For this review, take the finished solid that the model builds, in its own axes (mm). Round coordinates to 2 decimals unless told otherwise and drop trailing zeros. Order: outer loops, then holes, each group sorted by start corner. A loop starts at its lowest first (then second) coordinate and runs counter-clockwise, first axis right, second up. Notation, with made-up numbers: M -1,9.5 L 32,9.5 A28 cw 32,37.5 Z; hole C 48.5,45.25 d5. An arc over 180 degrees is marked long. Write item = value, one per line. Start each with the question number.
from build123d import *

# Parameters (mm, degrees)
F0_R     = 14.059963
F1_DEPTH = 30


with BuildPart() as f1:
    # F0 (on Front) → F1 (new body)
    with BuildSketch(Plane.XZ):
        with BuildLine():
            Line((28.253531, -42.646307), (28.253531, 42.646307))
            Line((28.253531, 42.646307), (27.968869, 42.646307))
            ThreePointArc((27.968869, 42.646307), (0, 70.615176), (-27.968869, 42.646307))
            Line((-27.968869, 42.646307), (-28.253531, 42.646307))
            Line((-28.253531, 42.646307), (-28.253531, -42.646307))
            Line((-28.253531, -42.646307), (28.253531, -42.646307))
        make_face()
        with Locations((0, 42.646307)):
            Circle(F0_R, mode=Mode.SUBTRACT)
    extrude(amount=F1_DEPTH)


solid = f1.part
(1) Insertion check: pin 1 (4 mm diameter, centred on x = -14.5, y = -12, fed in from +Z); pin 2 (3 mm diameter, centred on x = 0, z = 12, fed in from +Y); pin 3 (2 mm diameter, centred on x = 1, y = -8.5, fed in from +Z). Each pin has a flat end and moves straight along its axis. Give the tip position at first contact, or say it passes through.
(2) We need section C-C, the plane z = 37.5. Write out the cut boundary in (x, y).
(3) We need section D-D, the plane x = -19. Write out the cut boundary in (y, z).
(4) Draft analysis for pull direction X (two halves, no side actions). For faces 1 (the flat face through (0, -15, -42.646)), 2 (the flat face through (-28.254, -15, 1)), 3 (the cylindrical face through (-3.05, -14.79, 28.92)), 4 (the flat face through (28.254, -15, -1)), state which applies: released by +X, released by -X, zero draft, split by the parting line, or undercut.
(5) For line 1 along Z through (x, y) = (0, -8.5); line 2 along X through (y, z) = (-21.75, 42.5); line 3 along X through (y, z) = (-14, 43), list the stretches that pass through material, from the lowest coordinate up.
(6) We need section B-B, the plane y = -5. Write out the cut boundary in (x, z), then the cut area to 3 significant figures.
(7) We need section A-A, the plane x = 0. Write out the cut boundary in (y, z), then the cut area to 3 significant figures.
Values:
q1.pin_1 = 67.67
q1.pin_2 = 0
q1.pin_3 = 70.62
q2.outline = M -28.25,-30 L -13.08,-30 L -13.08,0 L -28.25,0 Z; M 13.08,-30 L 28.25,-30 L 28.25,0 L 13.08,0 Z
q3.outline = M -30,-42.65 L 0,-42.65 L 0,63.17 L -30,63.17 Z
q4.face_1 = zero draft
q4.face_2 = released by -X
q4.face_3 = undercut
q4.face_4 = released by +X
q5.line_1 = -42.65 to 28.59, 56.71 to 70.62
q5.line_2 = -28.25 to -14.06, 14.06 to 28.25
q5.line_3 = -27.97 to -14.06, 14.06 to 27.97
q6.outline = M -28.25,-42.65 L 28.25,-42.65 L 28.25,42.65 L 27.97,42.65 A27.97 ccw -27.97,42.65 L -28.25,42.65 Z; hole C 0,42.65 d28.12
q6.area = 5,430 mm²
q7.outline = M -30,-42.65 L 0,-42.65 L 0,28.59 L -30,28.59 Z; M -30,56.71 L 0,56.71 L 0,70.62 L -30,70.62 Z
q7.area = 2,550 mm²
